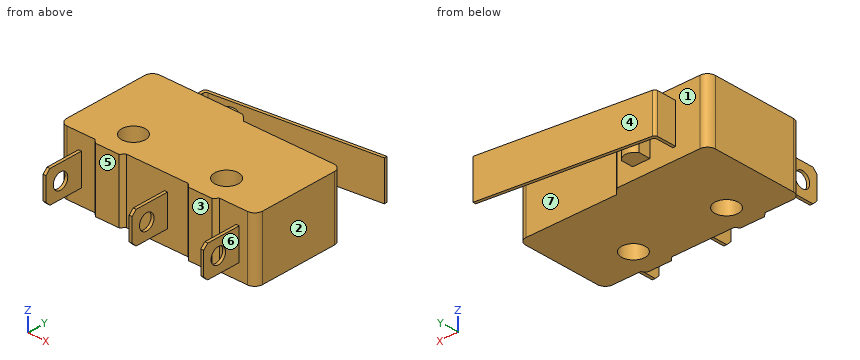
```python
from build123d import *

# Parameters (mm, degrees)
SKETCH1_W           = 20
SKETCH1_H           = 10.2
BOSS_EXTRUDE1_DEPTH = 6.4
SKETCH2_W           = 0.3
SKETCH2_H           = 3.2
BOSS_EXTRUDE2_DEPTH = 3.9
CUT_EXTRUDE1_REACH  = 23.163
SKETCH3_R           = 0.8
LPATTERN1_COUNT     = 2
LPATTERN1_PITCH     = 8.8
LPATTERN2_COUNT     = 2
LPATTERN2_PITCH     = 16.1
SKETCH4_W           = 10
SKETCH4_H           = 6.4
CUT_EXTRUDE2_DEPTH  = 0.7
SKETCH5_R           = 1.2
CUT_EXTRUDE3_DEPTH  = 15.898322053
BOSS_EXTRUDE3_DEPTH = 6.4
CHAMFER1_SIZE       = 0.7
FILLET1_R           = 0.8
BOSS_EXTRUDE4_START = -1.2
BOSS_EXTRUDE4_DEPTH = 4
BOSS_EXTRUDE5_DEPTH = 4
FILLET2_R           = 0.3


with BuildPart() as part:
    # Sketch1 → Boss-Extrude1 (new body)
    with BuildSketch(Plane.XY):
        Rectangle(SKETCH1_W, SKETCH1_H)
    extrude(amount=BOSS_EXTRUDE1_DEPTH)

    # Sketch2 → Boss-Extrude2 (add)
    with BuildSketch(Plane.XZ.offset(5.1)):
        with Locations((-7.902688508, 3.2)):
            Rectangle(SKETCH2_W, SKETCH2_H)
    boss_extrude2 = extrude(amount=BOSS_EXTRUDE2_DEPTH)

    # Sketch3 → Cut-Extrude1 (cut, up to next)
    with BuildSketch(Plane.ZY.offset(8.052688508), mode=Mode.PRIVATE) as cut_extrude1_sk1:
        with Locations((3.2, -7.395440134)):
            Circle(SKETCH3_R)
    cut_extrude1_tool1 = extrude(cut_extrude1_sk1.sketch, amount=-CUT_EXTRUDE1_REACH, mode=Mode.PRIVATE) & part.part
    # Sketch3 → Cut-Extrude1 (cut, up to next)
    with BuildSketch(Plane.ZY.offset(8.052688508), mode=Mode.PRIVATE) as cut_extrude1_sk2:
        Polygon((4.362215953, -9), (4.8, -8.562215953), (4.8, -9), align=None)
    cut_extrude1_tool2 = extrude(cut_extrude1_sk2.sketch, amount=-CUT_EXTRUDE1_REACH, mode=Mode.PRIVATE) & part.part
    # Sketch3 → Cut-Extrude1 (cut, up to next)
    with BuildSketch(Plane.ZY.offset(8.052688508), mode=Mode.PRIVATE) as cut_extrude1_sk3:
        Polygon((2.037784047, -9), (1.6, -8.562215953), (1.6, -9), align=None)
    cut_extrude1_tool3 = extrude(cut_extrude1_sk3.sketch, amount=-CUT_EXTRUDE1_REACH, mode=Mode.PRIVATE) & part.part
    cut_extrude1_1 = cut_extrude1_tool1.solids().sort_by_distance((-8.052689, -7.39544, 3.2))[0]
    add(cut_extrude1_1, mode=Mode.SUBTRACT)
    cut_extrude1_2 = cut_extrude1_tool2.solids().sort_by_distance((-8.052689, -8.854072, 4.654072))[0]
    add(cut_extrude1_2, mode=Mode.SUBTRACT)
    cut_extrude1_3 = cut_extrude1_tool3.solids().sort_by_distance((-8.052689, -8.854072, 1.745928))[0]
    add(cut_extrude1_3, mode=Mode.SUBTRACT)
    cut_extrude1 = cut_extrude1_1 + cut_extrude1_2 + cut_extrude1_3  # Cut-Extrude1 as one shape, for the pattern or mirror that repeats it

    # LPattern1: Boss-Extrude2, Cut-Extrude1 ×2
    with Locations(*[(i * LPATTERN1_PITCH, 0, 0) for i in range(1, LPATTERN1_COUNT)]):
        add(boss_extrude2)
        add(cut_extrude1, mode=Mode.SUBTRACT)

    # LPattern2: Boss-Extrude2, Cut-Extrude1 ×2
    with Locations(*[(i * LPATTERN2_PITCH, 0, 0) for i in range(1, LPATTERN2_COUNT)]):
        add(boss_extrude2)
        add(cut_extrude1, mode=Mode.SUBTRACT)

    # Sketch4 → Cut-Extrude2 (cut)
    with BuildSketch(Plane(origin=(0, 5.1, 0), x_dir=(1, 0, 0), z_dir=(0, 1, 0))):
        with Locations((5, -3.2)):
            Rectangle(SKETCH4_W, SKETCH4_H)
    extrude(amount=-CUT_EXTRUDE2_DEPTH, mode=Mode.SUBTRACT)

    # Sketch5 → Cut-Extrude3 (cut, through all)
    with BuildSketch(Plane.XY.offset(6.4)):
        with Locations((-4.75, -2.6)):
            Circle(SKETCH5_R)
        with Locations((4.75, -2.6)):
            Circle(SKETCH5_R)
    extrude(amount=-CUT_EXTRUDE3_DEPTH, mode=Mode.SUBTRACT)

    # Sketch7 → Boss-Extrude3 (add)
    with BuildSketch(Plane.XY.offset(6.4)):
        Polygon((-3.55, -5.5), (-5.95, -5.5), (-6.35, -5.1), (-3.15, -5.1), align=None)
        Polygon((5.95, -5.5), (3.55, -5.5), (3.15, -5.1), (6.35, -5.1), align=None)
    extrude(amount=-BOSS_EXTRUDE3_DEPTH)

    # Chamfer1
    chamfer1_edges = [part.edges().sort_by_distance(p)[0] for p in [
        (0, 5.1, 3.2),
    ]]
    chamfer(chamfer1_edges, length=CHAMFER1_SIZE - 0.0001)  # a hair under: the kernel refuses the full size

    # Fillet1
    fillet1_edges = [part.edges().sort_by_distance(p)[0] for p in [
        (10, 4.4, 3.2),
        (10, -5.1, 3.2),
        (-10, -5.1, 3.2),
        (-10, 5.1, 3.2),
    ]]
    fillet(fillet1_edges, radius=FILLET1_R)

    # Sketch8 → Boss-Extrude4 (add)
    with BuildSketch(Plane.XY.offset(6.4).offset(BOSS_EXTRUDE4_START)):
        with BuildLine():
            Line((-2.300370524, 5.1), (-2.300370524, 6.3))
            ThreePointArc((-2.300370524, 6.3), (-3.188470104, 6.802852397), (-4.076569683, 6.3))
            Line((-4.076569683, 6.3), (-4.076569683, 5.1))
            Line((-4.076569683, 5.1), (-2.300370524, 5.1))
        make_face()
    extrude(amount=-BOSS_EXTRUDE4_DEPTH)

    # Sketch11 → Boss-Extrude5 (add)
    with BuildSketch(Plane.XY.offset(5.2)):
        Polygon((-6.4, 5.1), (-6.7, 5.1), (-6.7, 7.349497833), (10, 9.4), (10, 9.097747052), (-6.4, 7.084080254), align=None)
    extrude(amount=-BOSS_EXTRUDE5_DEPTH)

    # Fillet2
    fillet2_edges = [part.edges().sort_by_distance(p)[0] for p in [
        (-6.7, 7.349497833, 3.2),
        (-6.4, 7.084080254, 3.2),
    ]]
    fillet(fillet2_edges, radius=FILLET2_R)


solid = part.part
```
Here's how the part is built. I have some questions about the finished solid (model axes, mm). Face numbers are marked on the shaded views. A direction names the side the tool comes from. Give positions to 0.01 mm unless a question says otherwise; leave off trailing zeros. Order: outer loops, then holes, each group sorted by start corner. A loop starts at its lowest first (then second) coordinate and runs counter-clockwise, first axis right, second up. Notation, with made-up numbers: (-22, 49.25) -> (13, 49.25) arc R6 ccw to (13, 55.25) -> close; hole circle Ø11 at (-1, 67.25). An arc over 180 degrees is marked (long way). Use CSV: the item, a comma, the result in double quotes. Start each with the question number.
Item 1: On a 3-axis mill with a long thin cutter (end or side, diameter ignored), from which of +Z, -Z, +X, -X, +Y, -Y can I reach the whole of each face in a straight line? I mean the marked faces 5, 6 and 7. Say none if no direction works.
Item 2: Thinking about a two-plate mould opening in Y: for the marked faces 1, 2, 3 and 4, which applies, pulls with the +Y half, pulls with the -Y half, needs draft (parallel to the pull), parting line crosses it, or undercut?
Item 3: Suppose I cut it at A-A (y = -2.6). List the corners of the cut face in (x, z) for me, and give its area (3 significant figures).
Item 4: Suppose I cut it at B-B (x = 4.5). List the corners of the cut face in (y, z) for me.
Item 5: Suppose I cut it at C-C (z = 3). Give the number of separate pieces and of enclosed holes in the cut face, and give its area (3 significant figures).
Item 6: I'm going to push flat-ended pins straight in: P1, Ø2, axis at y = -7.4, z = 3.2, coming from the +X side; P2, Ø1, axis at x = -0.5, z = 4.5, coming from the +Y side; P3, Ø2.5, axis at y = -7.4, z = 3.2, coming from the -X side; P4, Ø1.9, axis at x = 4.75, y = -2.6, coming from the -Z side. Where does each tip first touch, or does it pass through?
Item 7: If I drill on probe 1 along X at (y, z) = (-6.5, 4.5); probe 2 along X at (y, z) = (6, 5); probe 3 along Y at (x, z) = (4.75, 4.75), over which ranges is the centre line in solid material (lowest first)? Write a range as [from, to].
Answer block:
1,face 5,"+Z, -Z, -Y"
1,face 6,"+Z, -Z, +X, -Y"
1,face 7,"+Z, -Z, +X"
2,face 1,"undercut"
2,face 2,"needs draft"
2,face 3,"pulls with the -Y half"
2,face 4,"pulls with the +Y half"
3,outline,"(-10, 0) -> (-5.95, 0) -> (-5.95, 6.4) -> (-10, 6.4) -> close; (-3.55, 0) -> (3.55, 0) -> (3.55, 6.4) -> (-3.55, 6.4) -> close; (5.95, 0) -> (10, 0) -> (10, 6.4) -> (5.95, 6.4) -> close"
3,area,"97.3 mm^2"
4,outline,"(-5.5, 0) -> (-3.77, 0) -> (-3.77, 6.4) -> (-5.5, 6.4) -> close; (-1.43, 0) -> (4.4, 0) -> (4.4, 6.4) -> (-1.43, 6.4) -> close; (8.42, 1.2) -> (8.72, 1.2) -> (8.72, 5.2) -> (8.42, 5.2) -> close"
5,separate pieces,"4"
5,enclosed holes,"2"
5,area,"200 mm^2"
6,P1,"stops at x = 8.35"
6,P2,"stops at y = 8.17"
6,P3,"stops at x = -8.05"
6,P4,"passes through"
7,probe 1,"x = [-8.05, -7.75], [0.75, 1.05], [8.05, 8.35]"
7,probe 2,"x = [-6.7, -6.4], [-4.08, -2.3]"
7,probe 3,"y = [-5.5, -3.8], [-1.4, 4.4], [8.45, 8.76]"
